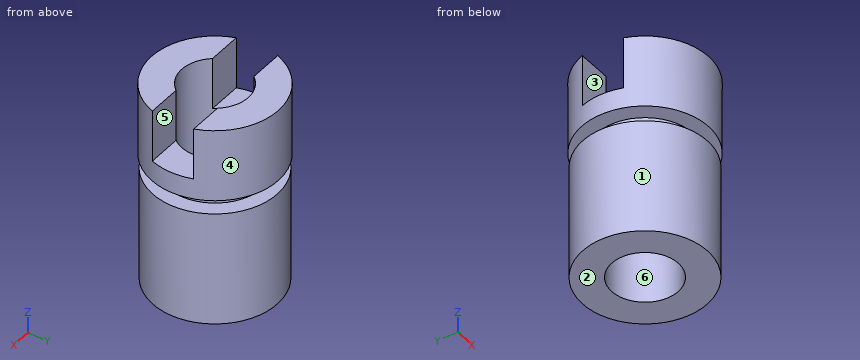
from build123d import *

# Parameters (mm, degrees)
SKETCH1_R           = 3
SKETCH1_R_2         = 1.6
BOSS_EXTRUDE1_DEPTH = 5.5
SKETCH2_R           = 2.3
SKETCH2_R_2         = 1.6
BOSS_EXTRUDE2_DEPTH = 0.7
SKETCH3_R           = 3.05
SKETCH3_R_2         = 2.3
SKETCH3_R_3         = 1.6
BOSS_EXTRUDE3_DEPTH = 3.5
SKETCH4_W           = 6.2
SKETCH4_H           = 2
CUT_EXTRUDE1_DEPTH  = 2.5


with BuildPart() as part:
    # Sketch1 → Boss-Extrude1 (new body)
    with BuildSketch(Plane.XY):
        Circle(SKETCH1_R)
        Circle(SKETCH1_R_2, mode=Mode.SUBTRACT)
    extrude(amount=BOSS_EXTRUDE1_DEPTH)

    # Sketch2 → Boss-Extrude2 (add)
    with BuildSketch(Plane.XY.offset(5.5)):
        Circle(SKETCH2_R)
        Circle(SKETCH2_R_2, mode=Mode.SUBTRACT)
    extrude(amount=BOSS_EXTRUDE2_DEPTH)

    # Sketch3 → Boss-Extrude3 (add)
    # profile 1 of 2: a face of its own
    with BuildSketch(Plane.XY.offset(6.2)):
        Circle(SKETCH3_R)
        Circle(SKETCH3_R_2, mode=Mode.SUBTRACT)
    # profile 2 of 2: a face of its own
    with BuildSketch(Plane.XY.offset(6.2)):
        Circle(SKETCH3_R_2)
        Circle(SKETCH3_R_3, mode=Mode.SUBTRACT)
    extrude(amount=BOSS_EXTRUDE3_DEPTH)

    # Sketch4 → Cut-Extrude1 (cut)
    with BuildSketch(Plane.XY.offset(9.7)):
        Rectangle(SKETCH4_W, SKETCH4_H)
    extrude(amount=-CUT_EXTRUDE1_DEPTH, mode=Mode.SUBTRACT)


solid = part.part
Geometry check sheet. Reference: the model listing, model coordinates, mm. Face numbers are marked on the shaded views. A direction names the side the tool comes from. Give positions to 0.01 mm unless a question says otherwise; leave off trailing zeros. Write each loop counter-clockwise with the first axis right and the second up, starting at its lowest first coordinate (ties: lowest second). Pieces come first, ordered by that corner, then holes.
1) Thickness scan on line 1 (Y direction, x = 0, z = 3.75); line 2 (X direction, y = 0, z = 6.75); line 3 (Z direction, x = -2, y = -2). Record the ranges inside material, lowest first.
Values follow:
line 1: y = -3 to -1.6, 1.6 to 3
line 2: x = -3.05 to -1.6, 1.6 to 3.05
line 3: z = 0 to 5.5, 6.2 to 9.7
2) Release check for a two-part mould opening along X. For the marked faces 4, 5 and 6 record: released by +X, released by -X, zero draft, split by the parting line, or undercut.
Values follow:
face 4: split by the parting line
face 5: zero draft
face 6: undercut
3) Set-up check for the marked faces 1, 2 and 3: record each of +Z, -Z, +X, -X, +Y, -Y from which the full face is reachable in a straight line by a thin tool's end or side.
Values follow:
face 1: -Z
face 2: -Z, +X, -X, +Y, -Y
face 3: +Z, +X, -X
4) Cross-section at D-D (z = 4). Record the boundary of the cut face in (x, y), plus the area to 3 significant figures.
Values follow:
outline: circle Ø6 at (0, 0); hole circle Ø3.2 at (0, 0)
area: 20.2 mm2
5) Go/stop test with flat-tipped pins: pin 1 Ø1.8 at (x, z) = (-2.5, 8) entering from +Y; pin 2 Ø1.8 at (x, z) = (-2.5, 9) entering from -Y; pin 3 Ø2 at (x, y) = (1, 0.5) entering from +Z; pin 4 Ø1 at (y, z) = (-1, 7) entering from +X. Record where each tip stops, or that it passes through.
Values follow:
pin 1: stops at y = 2.6
pin 2: stops at y = -2.6
pin 3: stops at z = 9.7
pin 4: stops at x = 3.01
6) Cross-section at A-A (y = 0). Record the boundary of the cut face in (x, z), plus the area to 3 significant figures.
Values follow:
outline: (-3.05, 6.2) - (-2.3, 6.2) - (-2.3, 5.5) - (-3, 5.5) - (-3, 0) - (-1.6, 0) - (-1.6, 7.2) - (-3.05, 7.2) - close; (1.6, 0) - (3, 0) - (3, 5.5) - (2.3, 5.5) - (2.3, 6.2) - (3.05, 6.2) - (3.05, 7.2) - (1.6, 7.2) - close
area: 19.3 mm2
7) Cross-section at C-C (x = 0). Record the boundary of the cut face in (y, z), plus the area to 3 significant figures.
Values follow:
outline: (-3.05, 6.2) - (-2.3, 6.2) - (-2.3, 5.5) - (-3, 5.5) - (-3, 0) - (-1.6, 0) - (-1.6, 9.7) - (-3.05, 9.7) - close; (1.6, 0) - (3, 0) - (3, 5.5) - (2.3, 5.5) - (2.3, 6.2) - (3.05, 6.2) - (3.05, 9.7) - (1.6, 9.7) - close
area: 26.5 mm2
8) Cross-section at B-B (z = 8.75). Record the boundary of the cut face in (x, y), plus the area to 3 significant figures.
Values follow:
outline: (-2.88, -1) arc R3.05 ccw to (2.88, -1) - (1.25, -1) arc R1.6 cw to (-1.25, -1) - close; (-2.88, 1) - (-1.25, 1) arc R1.6 cw to (1.25, 1) - (2.88, 1) arc R3.05 ccw to start
area: 15.2 mm2
